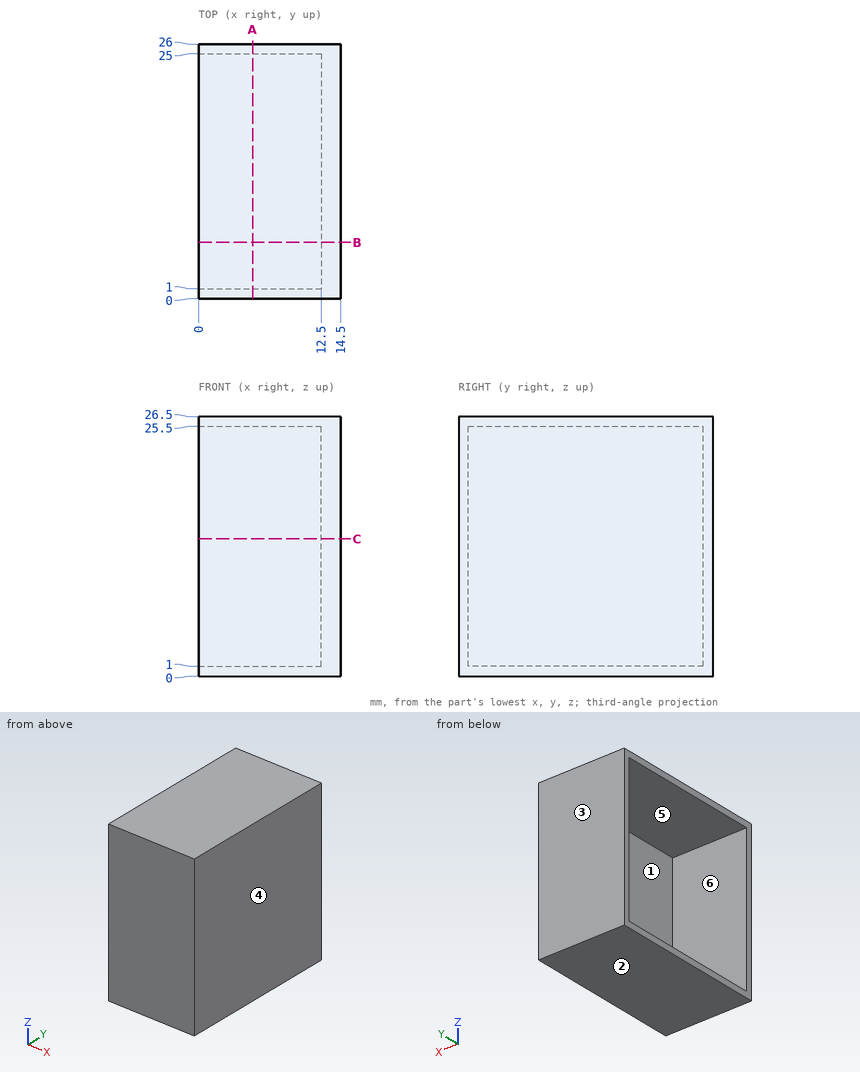
Could you check a few things on this drawing? It's one solid part, dimensions in mm from its lowest x, y, z. A direction names the side the tool comes from. Coordinates: 2 decimals unless noted, no trailing zeros. Loops run counter-clockwise (first coordinate to the right, second up) from the corner with the lowest first, then second, coordinate; pieces in that order, holes last. Notation, with made-up numbers: (6.5, -33.75) - (23.5, -33.75) arc R13 ccw to (23.5, -24.75) - close; hole circle Ø5 at (67, 49). An arc over 180 degrees is marked (long way). Answer as a JSON object with one key per item and string values. Group by question number.
Item 1: On a 3-axis mill with a long thin cutter (end or side, diameter ignored), from which of +Z, -Z, +X, -X, +Y, -Y can I reach the whole of each face in a straight line? I mean the marked faces 1 and 2. Say none if no direction works.
Item 2: If we mould it in two halves opening along Y, with no side actions, what happens to the marked faces 3, 4, 5 and 6? For each: released by +Y, released by -Y, zero draft, split by the parting line, or undercut.
Item 3: If we section it at C-C (z = 14): List the corners of the cut face in (x, y) for me.
Item 4: If we section it at B-B (y = 5.75): List the corners of the cut face in (x, z) for me.
Item 5: If I drill on L1, parallel to Z at x = 10, y = 23.25; L2, parallel to Y at x = 5, z = 11.5; L3, parallel to X at y = 10.75, z = 17.5, over which ranges is the centre line in solid material (lowest first)? Write a range as from..to.
Item 6: For pin 1 (4 mm diameter, centred on y = 12.5, z = 4, fed in from -X), with a flat end and sliding along its axis, tell me the tip position at first contact or that it passes through.
Item 7: If we section it at A-A (x = 5.5): List the corners of the cut face in (y, z) for me, plus the area to 3 significant figures.
Returned:
{
 "1": {"face 1": "-X", "face 2": "-Z, +X, -X, +Y, -Y"},
 "2": {"face 3": "released by +Y", "face 4": "zero draft", "face 5": "undercut", "face 6": "undercut"},
 "3": {"outline": "(0, 0) - (14.5, 0) - (14.5, 26) - (0, 26) - (0, 25) - (12.5, 25) - (12.5, 1) - (0, 1) - close"},
 "4": {"outline": "(0, 0) - (14.5, 0) - (14.5, 26.5) - (0, 26.5) - (0, 25.5) - (12.5, 25.5) - (12.5, 1) - (0, 1) - close"},
 "5": {"L1": "z = 0..1, 25.5..26.5", "L2": "y = 0..1, 25..26", "L3": "x = 12.5..14.5"},
 "6": {"pin 1": "stops at x = 12.5"},
 "7": {"outline": "(0, 0) - (26, 0) - (26, 26.5) - (0, 26.5) - close; hole (1, 1) - (25, 1) - (25, 25.5) - (1, 25.5) - close", "area": "101 mm²"}
}
